Design review of the part built by this model. Coordinates are the model's own, in mm. Coordinates: 2 decimals unless noted, no trailing zeros. Loops run counter-clockwise (first coordinate to the right, second up) from the corner with the lowest first, then second, coordinate; pieces in that order, holes last. Notation, with made-up numbers: (0.25, 74.25) -> (8.25, 74.25) arc R8 cw to (8.25, 87.25) -> close; hole circle Ø1 at (-30, -10). An arc over 180 degrees is marked (long way). Answer as a JSON object with one key per item and string values.
```python
from build123d import *

# Parameters (mm, degrees)
F0_W     = 4.5
F0_H     = 10
F1_DEPTH = 4.8


# Not quite as in the source:
# - a feature names something its author has since deleted; it is built from what else it names


with BuildPart() as f1:
    # F0 (on Front) → F1 (new body)
    with BuildSketch(Plane.XZ):
        Polygon((-167.476225, 0), (0, 0), (0, 15), (4.5, 15), (4.5, 25), (0, 25), (0, 45), (4.5, 45), (4.5, 55), (0, 55), (0, 70), (-172.276225, 70), (-182.276225, 70), (-344.95245, 70), (-344.95245, 55), (-349.45245, 55), (-349.45245, 45), (-344.95245, 45), (-344.95245, 25), (-344.95245, 15), (-344.95245, 0), (-177.476225, 0), align=None)
        Polygon((-167.476225, -0.2312080078), (-167.476225, 0), (-177.476225, 0), (-177.476225, -4.5), (-167.476225, -4.5), align=None)
        with Locations((-347.20245, 20)):
            Rectangle(F0_W, F0_H)
    extrude(amount=F1_DEPTH)


solid = f1.part
```
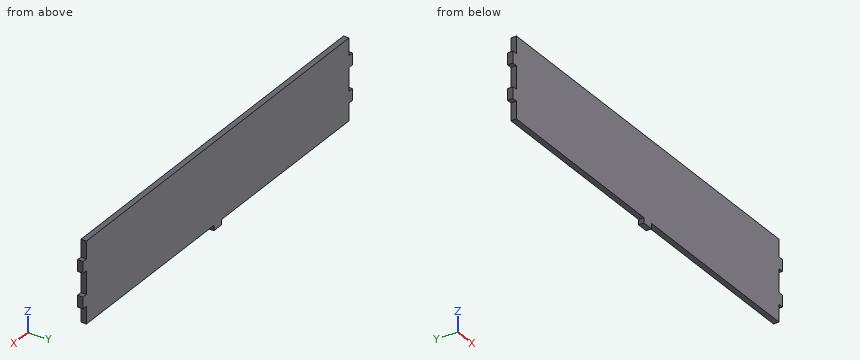
1) Add section B-B, the plane z = 36. Give the boundary of the cut face in (x, y).
Completed:
{"outline": "(-344.95, -4.8) -> (0, -4.8) -> (0, 0) -> (-344.95, 0) -> close"}
2) Clearance check with flat-ended pins moving along their axes: pin 1 Ø2 at (x, y) = (-143.5, -1.5) entering from -Z; pin 2 Ø2.5 at (y, z) = (-3.5, 4.5) entering from -X; pin 3 Ø1.4 at (y, z) = (-1.5, 63) entering from +X. State where each tip first meets the part, or that it passes through.
Completed:
{"pin 1": "z = 0", "pin 2": "x = -344.95", "pin 3": "x = 0"}
3) Wall thickness on probe 1 along Z at (x, y) = (-84.5, -0.9); probe 2 along X at (y, z) = (-3.45, 61): over which ranges is each line inside the solid? List them lowest first.
Completed:
{"probe 1": "0 to 70", "probe 2": "-344.95 to 0"}
4) Add section A-A, the plane y = -4. Give the boundary of the cut face in (x, z).
Completed:
{"outline": "(-349.45, 15) -> (-344.95, 15) -> (-344.95, 0) -> (-177.48, 0) -> (-177.48, -4.5) -> (-167.48, -4.5) -> (-167.48, 0) -> (0, 0) -> (0, 15) -> (4.5, 15) -> (4.5, 25) -> (0, 25) -> (0, 45) -> (4.5, 45) -> (4.5, 55) -> (0, 55) -> (0, 70) -> (-344.95, 70) -> (-344.95, 55) -> (-349.45, 55) -> (-349.45, 45) -> (-344.95, 45) -> (-344.95, 25) -> (-349.45, 25) -> close"}
5) Add section C-C, the plane x = -275. Give the boundary of the cut face in (y, z).
Completed:
{"outline": "(-4.8, 0) -> (0, 0) -> (0, 70) -> (-4.8, 70) -> close"}
